Read the model definition and answer for the solid it produces. Units are mm, in the model's axes. A direction names the side the tool comes from. Round coordinates to 2 decimals unless told otherwise and drop trailing zeros. Loops run counter-clockwise (first coordinate to the right, second up) from the corner with the lowest first, then second, coordinate; pieces in that order, holes last. Notation, with made-up numbers: M 62,47 L 118,47 A25 cw 118,66 Z; hole C -3.5,-10 d9. An arc over 180 degrees is marked long. Write each question's results on one line, items separated by ' | '.
```python
from build123d import *

# Parameters (mm, degrees)
SALIENTE_EXTRUIR1_DEPTH = 1.5
CROQUIS2_W              = 40
CROQUIS2_H              = 1.5
SALIENTE_EXTRUIR2_DEPTH = 41.5
CROQUIS3_R              = 1.5
CORTAR_EXTRUIR1_DEPTH   = 41.5
CROQUIS4_R              = 1.5
CORTAR_EXTRUIR2_DEPTH   = 41.5
FILLET1_R               = 3


with BuildPart() as part:
    # Croquis1 → Saliente-Extruir1 (new body)
    with BuildSketch(Plane.XY):
        with BuildLine():
            Line((0, 0), (40, 0))
            Line((40, 0), (40, 26))
            ThreePointArc((40, 26), (20, 46), (0, 26))
            Line((0, 26), (0, 0))
        make_face()
    extrude(amount=SALIENTE_EXTRUIR1_DEPTH)

    # Croquis2 → Saliente-Extruir2 (add)
    with BuildSketch(Plane.XY.offset(1.5)):
        with Locations((20, 0.75)):
            Rectangle(CROQUIS2_W, CROQUIS2_H)
    extrude(amount=SALIENTE_EXTRUIR2_DEPTH)

    # Croquis3 → Cortar-Extruir1 (cut)
    with BuildSketch(Plane(origin=(0, 1.5, 0), x_dir=(1, 0, 0), z_dir=(0, 1, 0))):
        with Locations(Location((5, -33.5, 0), (0, 0, 270))):
            Circle(CROQUIS3_R)
        with Locations(Location((5, -9.5, 0), (0, 0, 270))):
            Circle(CROQUIS3_R)
        with Locations(Location((35, -9.5, 0), (0, 0, 270))):
            Circle(CROQUIS3_R)
        with Locations(Location((35, -33.5, 0), (0, 0, 270))):
            Circle(CROQUIS3_R)
    extrude(amount=-CORTAR_EXTRUIR1_DEPTH, mode=Mode.SUBTRACT)

    # Croquis4 → Cortar-Extruir2 (cut)
    with BuildSketch(Plane.XY.offset(1.5)):
        with BuildLine():
            ThreePointArc((26.4, 33), (20, 39.4), (13.6, 33))
            Line((13.6, 33), (13.6, 19))
            ThreePointArc((13.6, 19), (20, 12.6), (26.4, 19))
            Line((26.4, 19), (26.4, 33))
        make_face()
        with Locations((12.25, 39.423393759)):
            Circle(CROQUIS4_R)
        with BuildLine():
            Line((13.749817566, 12.6), (13.6, 12.6))
            Line((13.6, 12.6), (13.6, 13.230441083))
            ThreePointArc((13.6, 13.230441083), (10.790640884, 12.229805189), (13.749817566, 12.6))
        make_face()
        with BuildLine():
            Line((26.250182434, 39.4), (26.4, 39.4))
            Line((26.4, 39.4), (26.4, 38.769558917))
            ThreePointArc((26.4, 38.769558917), (29.209359116, 39.770194811), (26.250182434, 39.4))
        make_face()
        with BuildLine():
            Line((26.4, 12.6), (26.250182434, 12.6))
            ThreePointArc((26.250182434, 12.6), (29.209359116, 12.229805189), (26.4, 13.230441083))
            Line((26.4, 13.230441083), (26.4, 12.6))
        make_face()
        with Locations((4.5, 26)):
            Circle(CROQUIS4_R)
        with Locations((35.5, 26)):
            Circle(CROQUIS4_R)
    extrude(amount=-CORTAR_EXTRUIR2_DEPTH, mode=Mode.SUBTRACT)

    # Fillet1
    fillet1_edges = [part.edges().sort_by_distance(p)[0] for p in [
        (0, 0.75, 43),
        (40, 0.75, 43),
    ]]
    fillet(fillet1_edges, radius=FILLET1_R)


solid = part.part
```
1. Given P1, Ø5, axis at x = 18.5, z = 24.5, coming from the +Y side; P2, Ø12, axis at x = 19, y = 23, coming from the +Z side; P3, Ø2.5, axis at x = 4.5, y = 26, coming from the +Z side, each flat-ended and moving along its own axis, determine where each tip first touches the part or whether it passes through.
Completed:
P1: stops at y = 1.5 | P2: stops at z = 1.5 | P3: passes through
2. Find section C-C, the plane y = 22.5. Give the vertices of the cut face in (x, z).
Completed:
outline: M 0,0 L 13.6,0 L 13.6,1.5 L 0,1.5 Z; M 26.4,0 L 40,0 L 40,1.5 L 26.4,1.5 Z
3. Determine the mould class of faces 1 (the face through (15, 13, 0)), 2 (the face through (20, 1.5, 22)), 3 (the face through (13.6, 26, 1)) for opening direction Y: released by +Y, released by -Y, zero draft, split by the parting line, or undercut.
Completed:
face 1: zero draft | face 2: released by +Y | face 3: undercut
4. Which of the six approach directions +Z, -Z, +X, -X, +Y, -Y give full straight-line access (tool end or side, diameter ignored) to faces 4 (the face through (20, 1, 43)), 5 (the face through (20.1, 39.4, 0.8)), 6 (the face through (15, 14, 1.5))?
Completed:
face 4: +Z, +X, -X, +Y, -Y | face 5: +Z, -Z | face 6: +Z, +X, -X, +Y
5. Find the intervals of material crossed by L1, parallel to Y at x = 27.75, z = 0.65; L2, parallel to Z at x = 32, y = 26.5, in increasing order.
Completed:
L1: y = 0 to 11.08, 14.08 to 37.92, 40.92 to 44.44 | L2: z = 0 to 1.5
6. Find section A-A, the plane x = 20. Give the vertices of the cut face in (y, z).
Completed:
outline: M 0,0 L 12.6,0 L 12.6,1.5 L 1.5,1.5 L 1.5,43 L 0,43 Z; M 39.4,0 L 46,0 L 46,1.5 L 39.4,1.5 Z
7. Find section B-B, the plane z = 33.5. Give the vertices of the cut face in (x, y), then the cut area to 3 significant figures.
Completed:
outline: M 0,0 L 3.5,0 L 3.5,1.5 L 0,1.5 Z; M 6.5,0 L 33.5,0 L 33.5,1.5 L 6.5,1.5 Z; M 36.5,0 L 40,0 L 40,1.5 L 36.5,1.5 Z | area: 51.0 mm2
8. Find section D-D, the plane x = 27.75. Give the vertices of the cut face in (y, z).
Completed:
outline: M 0,0 L 11.08,0 L 11.08,1.5 L 1.5,1.5 L 1.5,43 L 0,43 Z; M 14.08,0 L 37.92,0 L 37.92,1.5 L 14.08,1.5 Z; M 40.92,0 L 44.44,0 L 44.44,1.5 L 40.92,1.5 Z
